Autodesk Inventor part; units mm, degrees
ref_plane "YZ Plane" through (0, 0, 0) normal (1, 0, 0) x (0, 1, 0)
ref_plane "XZ Plane" through (0, 0, 0) normal (0, 1, 0) x (-1, 0, 0)
ref_plane "XY Plane" through (0, 0, 0) normal (0, 0, 1) x (1, 0, 0)
sketch "Sketch1" plane through (0, 0, 0) normal (0, 0, 1) x (1, 0, 0)
  line L0 (-75, -50) -> (75, -50)
  line L1 (75, -50) -> (75, 200)
  line L2 (75, 200) -> (-75, 200)
  line L3 (-75, 200) -> (-75, -50)
  circle A0 centre (0, 0) radius 20
  line L4 (0, 0) -> (0, 30) construction
  dimension "d0" = 150
  dimension "d1" = 250
  dimension "d2" = 40
  dimension "d16" = 30
  dimension "d17" = 50
extrude "Extrusion1" add sketch "Sketch1" along normal blind 6
hole "Hole1" at (0, 30, 0) direction (0, 0, 1) diameter 3 end through all
pattern_circular "Circular Pattern1" count 6 over 360 about axis through (0, 0, 0) along (0, 0, 1) of "Hole1"
properties part number "base_plate" material "Plywood, Finish"
Design review of the part built by this model. Coordinates are the model's own, in mm. Coordinates: 2 decimals unless noted, no trailing zeros. Write each loop counter-clockwise with the first axis right and the second up, starting at its lowest first coordinate (ties: lowest second). Pieces come first, ordered by that corner, then holes.
1) Add section A-A (y = 0). Write out the cut boundary in (x, z), plus the area to 3 significant figures.
2) Mouldability with a two-part tool opening along Y and no side actions: class faces 1 (the cylindrical face through (-4.336, 19.524, 2.958)), 2 (the flat face through (-1, 77, 6)), 3 (the flat face through (1, 200, 3)), 4 (the flat face through (-1, -50, 3)) as +Y half, -Y half, draft (parallel to the pull), parting line (faces both ways), or undercut.
3) Add section C-C (z = 2.7). Write out the cut boundary in (x, y), plus the area to 3 significant figures.
4) To check wall thickness, follow L1, parallel to Y at x = 26, z = 1.3; L2, parallel to X at y = -15, z = 3.1; L3, parallel to Y at x = 18, z = 4. State the ranges of each line that lie inside material, in increasing order.
5) Add section B-B (x = -10). Write out the cut boundary in (y, z), plus the area to 3 significant figures.
Check result:
1. outline: (-75, 0) - (-20, 0) - (-20, 6) - (-75, 6) - close; (20, 0) - (75, 0) - (75, 6) - (20, 6) - close
1. area: 660 mm2
2. face 1: undercut
2. face 2: draft
2. face 3: +Y half
2. face 4: -Y half
3. outline: (-75, -50) - (75, -50) - (75, 200) - (-75, 200) - close; hole circle Ø3 at (-25.98, -15); hole circle Ø3 at (-25.98, 15); hole circle Ø40 at (0, 0); hole circle Ø3 at (0, -30); hole circle Ø3 at (0, 30); hole circle Ø3 at (25.98, -15); hole circle Ø3 at (25.98, 15)
3. area: 36,200 mm2
4. L1: y = -50 to -16.5, -13.5 to 13.5, 16.5 to 200
4. L2: x = -75 to -27.48, -24.48 to -13.23, 13.23 to 24.48, 27.48 to 75
4. L3: y = -50 to -8.72, 8.72 to 200
5. outline: (-50, 0) - (-17.32, 0) - (-17.32, 6) - (-50, 6) - close; (17.32, 0) - (200, 0) - (200, 6) - (17.32, 6) - close
5. area: 1,290 mm2
